Read the model definition and answer for the solid it produces. Units are mm, in the model's axes. A direction names the side the tool comes from. Coordinates: 2 decimals unless noted, no trailing zeros. Order: outer loops, then holes, each group sorted by start corner. A loop starts at its lowest first (then second) coordinate and runs counter-clockwise, first axis right, second up.
Autodesk Inventor part; units mm, degrees
ref_plane "YZ Plane" through (0, 0, 0) normal (1, 0, 0) x (0, 1, 0)
ref_plane "XZ Plane" through (0, 0, 0) normal (0, 1, 0) x (-1, 0, 0)
ref_plane "XY Plane" through (0, 0, 0) normal (0, 0, 1) x (1, 0, 0)
sketch "Sketch1" plane through (0, 0, 0) normal (0, 1, 0) x (-1, 0, 0)
  circle A0 centre (0, 0) radius 1
  dimension "d0" = 2
extrude "Extrusion1" add sketch "Sketch1" along normal blind 14
sketch "Sketch2" plane through (0, 0, 0) normal (0, -1, 0) x (1, 0, 0)
  circle A0 centre (0, 0) radius 2.5
extrude "Extrusion2" add sketch "Sketch2" along normal blind 1.5
fillet "Fillet1" radius 0.5 2 edges at (-2.5, -1.5, 0) (-2.5, 0, 0)
sketch "Sketch3" plane through (0, -1.5, 0) normal (0, -1, 0) x (1, 0, 0)
  line L0 (1.75, -0.5) -> (1.75, 0.5)
  line L1 (-1.75, 0.5) -> (-1.75, -0.5)
  line L2 (0.5, 1.75) -> (-0.5, 1.75)
  line L3 (-0.5, -1.75) -> (0.5, -1.75)
  line L4 (1.75, 0.5) -> (0.866, 0.5)
  line L5 (-0.866, 0.5) -> (-1.75, 0.5)
  line L6 (-0.5, 1.75) -> (-0.5, 0.866)
  line L7 (-0.5, -0.866) -> (-0.5, -1.75)
  line L8 (0.5, 0.866) -> (0.5, 1.75)
  line L9 (-1.75, -0.5) -> (-0.866, -0.5)
  line L10 (0.866, -0.5) -> (1.75, -0.5)
  line L11 (0.5, -1.75) -> (0.5, -0.866)
  arc A0 (-0.5, 0.866) -> (-0.866, 0.5) centre (0, 0) ccw
  arc A1 (0.866, 0.5) -> (0.5, 0.866) centre (0, 0) ccw
  arc A2 (-0.866, -0.5) -> (-0.5, -0.866) centre (0, 0) ccw
  arc A3 (0.5, -0.866) -> (0.866, -0.5) centre (0, 0) ccw
extrude "Extrusion3" cut sketch "Sketch3" against normal blind 1.2
chamfer "Chamfer1" distance 1 angle 45 1 edges at (1, 14, 0)
thread "Thread1"
properties part number "parafuso interno da ponte"
1) Determine the mould class of faces 1 (the flat face through (1, -1.5, -1)), 2 (the flat face through (1.3, -0.9, -0.5)), 3 (the cylindrical face through (0, 6, 1)) for opening direction Z: pulls with the +Z half, pulls with the -Z half, needs draft (parallel to the pull), parting line crosses it, or undercut.
A:
face 1: needs draft
face 2: undercut
face 3: parting line crosses it
2) Which of the six approach directions +Z, -Z, +X, -X, +Y, -Y give full straight-line access (tool end or side, diameter ignored) to faces 4 (the flat face through (0, -1, 1.75)), 5 (the flat face through (1, 0, -1)), 6 (the cylindrical face through (-0.54, -0.75, 2.44))?
A:
face 4: -Y
face 5: +Y
face 6: +Y, -Y
3) Flat-ended cylindrical pins translate along their axes: pin 1 Ø1 at (x, y) = (-1.5, -0.5) entering from +Z; pin 2 Ø2 at (x, z) = (1, -0.5) entering from +Y; pin 3 Ø0.7 at (y, z) = (-0.5, -1.5) entering from +X; pin 4 Ø1 at (y, z) = (9.5, 2) entering from -X. Find the tip coordinate at first contact, or state that the pin passes through.
A:
pin 1: stops at z = 2.29
pin 2: stops at y = 13.88
pin 3: stops at x = 2.22
pin 4: passes through
4) A cutting plane is placed at A-A, the plane y = 7. Determine the outline of the cut face in (x, z).
A:
outline: circle Ø2 at (0, 0)
5) Straight lines are drawn through the part: line 1 (Y direction, x = -1.05, z = 0.15); line 2 (Y direction, x = -0.4, z = 1.85); line 3 (Z direction, x = 0.25, y = 3.75). For each, find the intervals that lie inside material, in ascending order.
A:
line 1: y = -0.3 to 0
line 2: y = -1.5 to 0
line 3: z = -0.97 to 0.97
